Here's how the part is built. I have some questions about the finished solid (model axes, mm). A direction names the side the tool comes from. Round coordinates to 2 decimals unless told otherwise and drop trailing zeros. Write each loop counter-clockwise with the first axis right and the second up, starting at its lowest first coordinate (ties: lowest second). Pieces come first, ordered by that corner, then holes. Notation, with made-up numbers: (72, 43) -> (117, 43) arc R15 cw to (117, 69) -> close; hole circle Ø5 at (17.25, -18.75). An arc over 180 degrees is marked (long way). Answer in a Markdown table with one row per item. Add a question column.
from build123d import *

# Parameters (mm, degrees)
SM_BASE_FLANGE_1_DEPTH   = 25
CUT_EXTRUDE_1_DEPTH      = 46.365184889
CUT_EXTRUDE_1_DEPTH_BACK = 46.365184889
SKETCH_6_R               = 1.65
CUT_EXTRUDE_2_DEPTH      = 10
FILLET_1_R               = 2


# Sheet-metal steps are written as plain solids
with BuildPart() as part:
    # Sketch 1 → 基体-法兰1 (new, symmetric)
    with BuildSketch(Plane.XY):
        with BuildLine():
            Line((-36, 8), (-36, 1))
            ThreePointArc((-36, 1), (-35.707106781, 0.292893219), (-35, 0))
            Line((-35, 0), (35, 0))
            ThreePointArc((35, 0), (35.707106781, 0.292893219), (36, 1))
            Line((36, 1), (36, 8))
            Line((36, 8), (37, 8))
            Line((37, 8), (37, 1))
            ThreePointArc((37, 1), (36.414213562, -0.414213562), (35, -1))
            Line((35, -1), (-35, -1))
            ThreePointArc((-35, -1), (-36.414213562, -0.414213562), (-37, 1))
            Line((-37, 1), (-37, 8))
            Line((-37, 8), (-36, 8))
        make_face()
    extrude(amount=SM_BASE_FLANGE_1_DEPTH, both=True)

    # 草图6 → 切除-拉伸1 (cut, two sides: drawn at the far end of the back side and taken through both)
    with BuildSketch(Plane(origin=(0, 0, 0), x_dir=(0, 0, -1), z_dir=(1, 0, 0)).offset(-CUT_EXTRUDE_1_DEPTH_BACK)):
        with Locations((-20, 4.5)):
            Circle(SKETCH_6_R)
        with Locations((20, 4.5)):
            Circle(SKETCH_6_R)
        with BuildLine():
            Line((-13, 6.5), (13, 6.5))
            ThreePointArc((13, 6.5), (15, 4.5), (13, 2.5))
            Line((13, 2.5), (-13, 2.5))
            ThreePointArc((-13, 2.5), (-15, 4.5), (-13, 6.5))
        make_face()
    extrude(amount=CUT_EXTRUDE_1_DEPTH + CUT_EXTRUDE_1_DEPTH_BACK, mode=Mode.SUBTRACT)

    # 草图7 → 切除-拉伸2 (cut)
    with BuildSketch(Plane.XZ.offset(1)):
        with BuildLine():
            Line((-22, 15), (-22, -15))
            ThreePointArc((-22, -15), (-27, -20), (-32, -15))
            Line((-32, -15), (-32, 15))
            ThreePointArc((-32, 15), (-27, 20), (-22, 15))
        make_face()
        with BuildLine():
            Line((-8.5, 15), (-8.5, -15))
            ThreePointArc((-8.5, -15), (-13.5, -20), (-18.5, -15))
            Line((-18.5, -15), (-18.5, 15))
            ThreePointArc((-18.5, 15), (-13.5, 20), (-8.5, 15))
        make_face()
        with BuildLine():
            Line((5, 15), (5, -15))
            ThreePointArc((5, -15), (0, -20), (-5, -15))
            Line((-5, -15), (-5, 15))
            ThreePointArc((-5, 15), (0, 20), (5, 15))
        make_face()
        with BuildLine():
            Line((18.5, 15), (18.5, -15))
            ThreePointArc((18.5, -15), (13.5, -20), (8.5, -15))
            Line((8.5, -15), (8.5, 15))
            ThreePointArc((8.5, 15), (13.5, 20), (18.5, 15))
        make_face()
        with BuildLine():
            Line((32, 15), (32, -15))
            ThreePointArc((32, -15), (27, -20), (22, -15))
            Line((22, -15), (22, 15))
            ThreePointArc((22, 15), (27, 20), (32, 15))
        make_face()
    extrude(amount=-CUT_EXTRUDE_2_DEPTH, mode=Mode.SUBTRACT)

    # 圆角1
    fillet_1_edges = [part.edges().sort_by_distance(p)[0] for p in [
        (-36.5, 8, -25),
        (36.5, 8, -25),
        (-36.5, 8, 25),
        (36.5, 8, 25),
    ]]
    fillet(fillet_1_edges, radius=FILLET_1_R)


solid = part.part
Item 1: If we mould it in two halves opening along Y, with no side actions, what happens to faces 1 (the cylindrical face through (36.5, 4.5, 15)), 2 (the cylindrical face through (36.43, -0.4, 0.35)), 3 (the flat face through (36, 2, 0))? For each: pulls with the +Y half, pulls with the -Y half, needs draft (parallel to the pull), parting line crosses it, or undercut.
Item 2: I need wall thicknesses on line 1 along Z through (x, y) = (36.75, 4.5); line 2 along X through (y, z) = (6.75, -9); line 3 along X through (y, z) = (-0.5, -14). Which ranges of each line are inside material? Lowest first, please. Write a range as from..to.
Item 3: On a 3-axis mill with a long thin cutter (end or side, diameter ignored), from which of +Z, -Z, +X, -X, +Y, -Y can I reach the whole of each face in a straight line? I mean faces 4 (the flat face through (-36, 7, 0)), 5 (the cylindrical face through (-36.5, 4.5, -15)), 6 (the cylindrical face through (27.1, -0.5, -20)). Say none if no direction works.
Item 4: For P1, Ø25, axis at x = 1.5, z = 6, coming from the +Y side; P2, Ø0.8, axis at y = -0.5, z = 2, coming from the +X side; P3, Ø0.8, axis at y = -0.5, z = -5.5, coming from the -X side, each with a flat end and sliding along its axis, tell me the tip position at first contact or that it passes through.
Item 5: If we section it at C-C on x = -4: Please give me the cut outline in (y, z), then the cut area to 3 significant figures.
Item 6: If we section it at A-A on x = 13.5: Please give me the cut outline in (y, z), then the cut area to 3 significant figures.
Item 7: If we section it at B-B on y = 4.5: Give the number of separate pieces and of enclosed holes in the cut face, then the cut area to 3 significant figures.
Results list:
| question | item | result |
|---|---|---|
| 1 | face 1 | undercut |
| 1 | face 2 | pulls with the -Y half |
| 1 | face 3 | needs draft |
| 2 | line 1 | -25..-21.65, -18.35..-15, 15..18.35, 21.65..25 |
| 2 | line 2 | -37..-36, 36..37 |
| 2 | line 3 | -36.32..-32, -22..-18.5, -8.5..-5, 5..8.5, 18.5..22, 32..36.32 |
| 3 | face 4 | +Z, -Z, +Y |
| 3 | face 5 | +X, -X |
| 3 | face 6 | +Y, -Y |
| 4 | P1 | y = 0 |
| 4 | P2 | x = 36.67 |
| 4 | P3 | x = -36.67 |
| 5 | outline | (-1, -25) -> (0, -25) -> (0, -18) -> (-1, -18) -> close; (-1, 18) -> (0, 18) -> (0, 25) -> (-1, 25) -> close |
| 5 | area | 14.0 mm² |
| 6 | outline | (-1, -25) -> (0, -25) -> (0, -20) -> (-1, -20) -> close; (-1, 20) -> (0, 20) -> (0, 25) -> (-1, 25) -> close |
| 6 | area | 10.0 mm² |
| 7 | separate pieces | 8 |
| 7 | enclosed holes | 0 |
| 7 | area | 26.8 mm² |
